from build123d import *

# Parameters (mm, degrees)
SKETCH1_W                  = 17.5
SKETCH1_H                  = 35
BOSS_EXTRUDE1_DEPTH        = 97
M5_TAPPED_HOLE1_AT_2_COUNT = 2
M5_TAPPED_HOLE1_AT_2_PITCH = 20


with BuildPart() as part:
    # Sketch1 → Boss-Extrude1 (new, symmetric)
    with BuildSketch(Plane.XY):
        Rectangle(SKETCH1_W, SKETCH1_H)
    extrude(amount=BOSS_EXTRUDE1_DEPTH, both=True)

    # Sketch5 → M5 Tapped Hole1 (revolve, cut)
    with BuildSketch(Plane(origin=(0, 10, -97), x_dir=(0, 1, 0), z_dir=(1, 0, 0))):
        Polygon((0, 0), (0, 15.2618073), (2.1, 14), (2.1, 0.425), (2.525, 0), align=None)
    m5_tapped_hole1 = revolve(axis=Axis((0, 10, -103.35), (0, 0, 1)), mode=Mode.SUBTRACT)

    # M5 Tapped Hole1 at 2: M5 Tapped Hole1 ×2
    with Locations(*[(0, -i * M5_TAPPED_HOLE1_AT_2_PITCH, 0) for i in range(1, M5_TAPPED_HOLE1_AT_2_COUNT)]):
        add(m5_tapped_hole1, mode=Mode.SUBTRACT)

    # Mirror1: M5 Tapped Hole1 across plane
    add(m5_tapped_hole1.mirror(Plane.XY), mode=Mode.SUBTRACT)

    # Mirror1 copy 1 sketch → Mirror1 copy 1 (revolve, cut)
    with BuildSketch(Plane(origin=(0, -10, 97), x_dir=(0, 1, 0), z_dir=(1, 0, 0))):
        Polygon((0, 0), (0, -15.2618073), (2.1, -14), (2.1, -0.425), (2.525, 0), align=None)
    revolve(axis=Axis((0, -10, 103.35), (0, 0, 1)), mode=Mode.SUBTRACT)


solid = part.part
CAD build for the part. Positions are in the model's coordinates, mm. A direction names the side the tool comes from. Round coordinates to 2 decimals unless told otherwise and drop trailing zeros. Put each result on its own line as item: value. Start each with the question number.
1) 3-axis set-ups, long thin cutter, end or side, ignore diameter. For faces 1 (the cylindrical face through (-0.09, -12.1, -89.88)), 2 (the cylindrical face through (-0.09, -12.1, 89.88)), 3 (the flat face through (0, 17.5, 1)): which of +Z, -Z, +X, -X, +Y, -Y reach the whole face in a straight line?
2) Pull direction X, two halves, no side cores. Call faces 4 (the cylindrical face through (-0.09, 7.9, 89.88)), 5 (the flat face through (0, 0, 97)), 6 (the cylindrical face through (-0.09, 7.9, -89.88)), 7 (the flat face through (-8.75, 0, 1)): pulls with the +X half, pulls with the -X half, needs draft (parallel to the pull), parting line crosses it, or undercut.
3) Pin check, flat tips, straight feed: pin 1 Ø4 at (x, y) = (0, -10) entering from +Z; pin 2 Ø5 at (x, y) = (0, 10) entering from -Z (3 decimals). Stop position of each tip, or through.
4) Drill centre lines: probe 1 along Y at (x, z) = (0, 91.75); probe 2 along X at (y, z) = (10, 90); probe 3 along X at (y, z) = (-9.5, -85.5). Where is each one in solid material? Low to high. Write a range as [from, to].
Resolved:
1. face 1: -Z
1. face 2: +Z
1. face 3: +Z, -Z, +X, -X, +Y
2. face 4: undercut
2. face 5: needs draft
2. face 6: undercut
2. face 7: pulls with the -X half
3. pin 1: z = 82.94
3. pin 2: z = -96.975
4. probe 1: [-17.5, -12.1], [-7.9, 7.9], [12.1, 17.5]
4. probe 2: [-8.75, -2.1], [2.1, 8.75]
4. probe 3: [-8.75, -2.04], [2.04, 8.75]
